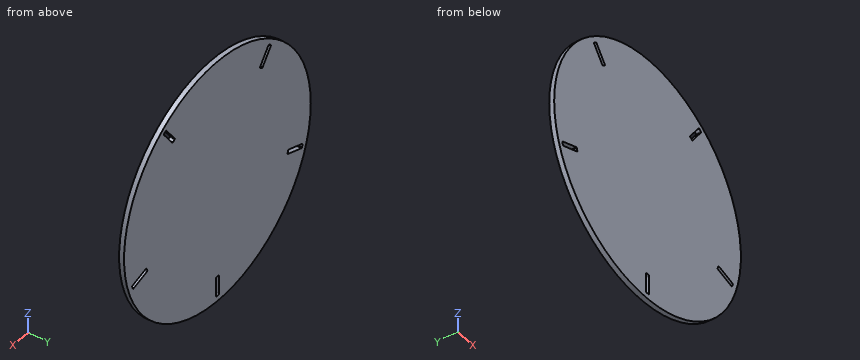
Autodesk Inventor part; units mm, degrees
ref_plane "YZ Plane" through (0, 0, 0) normal (1, 0, 0) x (0, 1, 0)
ref_plane "XZ Plane" through (0, 0, 0) normal (0, 1, 0) x (-1, 0, 0)
ref_plane "XY Plane" through (0, 0, 0) normal (0, 0, 1) x (1, 0, 0)
sketch "Sketch1" plane through (0, 0, 0) normal (0, 1, 0) x (-1, 0, 0)
  circle A0 centre (0, 0) radius 200
  dimension "d0" = 400
extrude "Extrusion1" add sketch "Sketch1" along normal blind 8
sketch "Sketch2" plane through (0, 8, 0) normal (0, 1, 0) x (1, 0, 0)
  line L0 (-1.9167, 191.4) -> (1.9167, 191.4)
  line L1 (3.25, 190.0667) -> (3.25, 160.0667)
  line L2 (1.9167, 158.7333) -> (-1.9167, 158.7333)
  line L3 (-3.25, 160.0667) -> (-3.25, 190.0667)
  circle A0 centre (0, 0) radius 200
  arc A1 (-1.9167, 191.4) -> (-3.25, 190.0667) centre (-1.9167, 190.0667) ccw
  arc A2 (3.25, 190.0667) -> (1.9167, 191.4) centre (1.9167, 190.0667) ccw
  arc A3 (1.9167, 158.7333) -> (3.25, 160.0667) centre (1.9167, 160.0667) ccw
  arc A4 (-3.25, 160.0667) -> (-1.9167, 158.7333) centre (-1.9167, 160.0667) ccw
  line L4 (114.1741, -153.6311) -> (111.0728, -155.8843)
  line L5 (109.2104, -155.5893) -> (91.5769, -131.3188)
  line L6 (91.8718, -129.4564) -> (94.9731, -127.2032)
  line L7 (96.8355, -127.4982) -> (114.469, -151.7687)
  arc A5 (114.1741, -153.6311) -> (114.469, -151.7687) centre (113.3904, -152.5524) ccw
  arc A6 (109.2104, -155.5893) -> (111.0728, -155.8843) centre (110.2891, -154.8056) ccw
  arc A7 (91.8718, -129.4564) -> (91.5769, -131.3188) centre (92.6556, -130.5351) ccw
  arc A8 (96.8355, -127.4982) -> (94.9731, -127.2032) centre (95.7568, -128.2819) ccw
  line L8 (181.3689, 61.1875) -> (182.5534, 57.5417)
  line L9 (181.6974, 55.8616) -> (153.1657, 46.5911)
  line L10 (151.4856, 47.4472) -> (150.301, 51.0929)
  line L11 (151.1571, 52.773) -> (179.6888, 62.0435)
  arc A9 (181.3689, 61.1875) -> (179.6888, 62.0435) centre (180.1008, 60.7754) ccw
  arc A10 (181.6974, 55.8616) -> (182.5534, 57.5417) centre (181.2854, 57.1297) ccw
  arc A11 (151.4856, 47.4472) -> (153.1657, 46.5911) centre (152.7537, 47.8592) ccw
  arc A12 (151.1571, 52.773) -> (150.301, 51.0929) centre (151.5691, 51.5049) ccw
  line L12 (-114.1741, -153.6311) -> (-111.0728, -155.8843)
  line L13 (-109.2104, -155.5893) -> (-91.5769, -131.3188)
  line L14 (-91.8718, -129.4564) -> (-94.9731, -127.2032)
  line L15 (-96.8355, -127.4982) -> (-114.469, -151.7687)
  arc A13 (-114.469, -151.7687) -> (-114.1741, -153.6311) centre (-113.3904, -152.5524) ccw
  arc A14 (-111.0728, -155.8843) -> (-109.2104, -155.5893) centre (-110.2891, -154.8056) ccw
  arc A15 (-91.5769, -131.3188) -> (-91.8718, -129.4564) centre (-92.6556, -130.5351) ccw
  arc A16 (-94.9731, -127.2032) -> (-96.8355, -127.4982) centre (-95.7568, -128.2819) ccw
  line L16 (-181.3689, 61.1875) -> (-182.5534, 57.5417)
  line L17 (-181.6974, 55.8616) -> (-153.1657, 46.5911)
  line L18 (-151.4856, 47.4472) -> (-150.301, 51.0929)
  line L19 (-151.1571, 52.773) -> (-179.6888, 62.0435)
  arc A17 (-179.6888, 62.0435) -> (-181.3689, 61.1875) centre (-180.1008, 60.7754) ccw
  arc A18 (-182.5534, 57.5417) -> (-181.6974, 55.8616) centre (-181.2854, 57.1297) ccw
  arc A19 (-153.1657, 46.5911) -> (-151.4856, 47.4472) centre (-152.7537, 47.8592) ccw
  arc A20 (-150.301, 51.0929) -> (-151.1571, 52.773) centre (-151.5691, 51.5049) ccw
  dimension "d3" = 191.4
  dimension "d4" = 6.5
  dimension "d6" = 1.3333
  dimension "d7" = 30
extrude "Extrusion2" cut sketch "Sketch2" against normal through all contours L0 A2 L1 A3 L2 A4 L3 A1 | L4 A6 L5 A7 L6 A8 L7 A5 | L8 A10 L9 A11 L10 A12 L11 A9 | A13 L15 A16 L14 A15 L13 A14 L12 | A17 L19 A20 L18 A19 L17 A18 L16
equation "\"BendRadius\" = Thickness"
equation "\"BendReliefWidth\" = Thickness"
equation "\"BendReliefDepth\" = 0.5 * Thickness"
equation "\"CornerReliefSize\" = 4 * Thickness"
equation "\"MinimumRemnant\" = 2 * Thickness"
equation "\"TransitionRadius\" = BendRadius"
equation "\"JacobiRadiusSize\" = BendRadius"
equation "\"GapSize\" = Thickness"
properties part number "fINAL Roof - G" material "Wood (Maple)"
Read the model definition and answer for the solid it produces. Units are mm, in the model's axes. Round coordinates to 2 decimals unless told otherwise and drop trailing zeros. Write each loop counter-clockwise with the first axis right and the second up, starting at its lowest first coordinate (ties: lowest second). Pieces come first, ordered by that corner, then holes. Notation, with made-up numbers: (11, 81) - (44, 81) arc R22 ccw to (44, 89) - close; hole circle Ø6 at (60, 87.25). An arc over 180 degrees is marked (long way). One line per item, written item: value.
Q1. Find section D-D (z = -143). Determine the outline of the cut face in (x, y), and give its area (3 significant figures).
The answers:
outline: (-139.82, 0) - (139.82, 0) - (139.82, 8) - (-139.82, 8) - close
area: 2,240 mm2
Q2. Each of these flat-tipped pins is pushed along its axis until it touches: P1, Ø2, axis at y = 6, z = -58.5, coming from the +X side; P2, Ø4, axis at y = 3.5, z = -171, coming from the -X side; P3, Ø4, axis at x = -153, y = 4, coming from the +Z side. Where does it stop, or does it pass through?
The answers:
P1: stops at x = 191.56
P2: stops at x = -106.95
P3: stops at z = 131.14
Q3. Find section B-B (y = 5.5). Count the separate pieces of the cut face and the enclosed holes in it, and give its area (3 significant figures).
The answers:
separate pieces: 1
enclosed holes: 5
area: 125,000 mm2
Q4. Find section C-C (z = -82). Determine the outline of the cut face in (x, y).
The answers:
outline: (-182.42, 0) - (182.42, 0) - (182.42, 8) - (-182.42, 8) - close
Q5. Straight lines are drawn through the part: line 1 (Z direction, x = -99, y = 4); line 2 (Z direction, x = -84.5, y = 4.5); line 3 (X direction, y = 4, z = -165). For each, find the intervals that lie inside material, in ascending order. Write a range as from..to.
The answers:
line 1: z = -173.78..130.48, 141.54..173.78
line 2: z = -181.27..181.27
line 3: x = -113.03..-3.25, 3.25..113.03
Q6. Find section A-A (x = -168). Determine the outline of the cut face in (y, z), and give its area (3 significant figures).
The answers:
outline: (0, -108.52) - (8, -108.52) - (8, -58.25) - (0, -58.25) - close; (0, -51.41) - (8, -51.41) - (8, 108.52) - (0, 108.52) - close
area: 1,680 mm2
